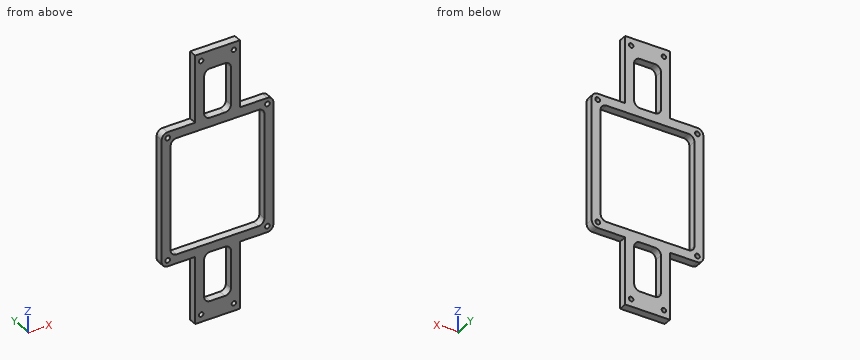
Autodesk Inventor part; units mm, degrees
ref_plane "YZ Plane" through (0, 0, 0) normal (1, 0, 0) x (0, 1, 0)
ref_plane "XZ Plane" through (0, 0, 0) normal (0, 1, 0) x (-1, 0, 0)
ref_plane "XY Plane" through (0, 0, 0) normal (0, 0, 1) x (1, 0, 0)
sketch "Sketch1" plane through (0, 0, 0) normal (0, 1, 0) x (-1, 0, 0)
  line L0 (37.5, 45) -> (-37.5, 45)
  line L1 (-37.5, 45) -> (-37.5, -45)
  line L2 (-37.5, -45) -> (37.5, -45)
  line L3 (37.5, -45) -> (37.5, 45)
  point P0 (0, 0)
  point P1 (37.5, 0)
  point P2 (0, 45)
  dimension "d0" = 90
  dimension "d1" = 75
extrude "Extrusion1" add sketch "Sketch1" along normal blind 5.334
sketch "Sketch2" plane through (0, 5.334, 0) normal (0, 1, 0) x (1, 0, 0)
  line L0 (-31.5, -39) -> (31.5, -39)
  line L1 (31.5, -39) -> (31.5, 39)
  line L2 (31.5, 39) -> (-31.5, 39)
  line L3 (-31.5, 39) -> (-31.5, -39)
  line L4 (-37.5, -45) -> (37.5, -45)
  line L5 (37.5, 45) -> (-37.5, 45)
  line L6 (-37.5, 45) -> (-37.5, -45)
  line L7 (37.5, -45) -> (37.5, 45)
  point P0 (0, 0)
  dimension "d4" = 6
  dimension "d5" = 6
  dimension "d6" = 6
  dimension "d7" = 6
extrude "Extrusion2" cut sketch "Sketch2" against normal through all contours L3 L2 L1 L0
sketch "Sketch3" plane through (0, 5.334, 0) normal (0, 1, 0) x (1, 0, 0)
  line L0 (-37.5, -45) -> (37.5, -45)
  line L1 (-37.5, 45) -> (-37.5, -45)
  line L2 (37.5, -45) -> (37.5, 45)
  line L3 (37.5, 45) -> (-37.5, 45)
  point P0 (0, 0)
  point P1 (-33.5, -41)
  point P2 (-33.5, 41)
  point P3 (33.5, 41)
  point P4 (33.5, -41)
  dimension "d10" = 4
  dimension "d11" = 4
  dimension "d12" = 4
  dimension "d13" = 4
hole "Hole1" at (-33.5, 5.334, 41) at (-33.5, 5.334, -41) at (33.5, 5.334, -41) at (33.5, 5.334, 41) direction (0, -1, 0) diameter 3.2 end through all
fillet "Fillet1" radius 4 8 edges at (-37.5, 2.667, 45) (-31.5, 2.667, 39) (37.5, 2.667, 45) (37.5, 2.667, -45) (31.5, 2.667, -39) (31.5, 2.667, 39) (-31.5, 2.667, -39) (-37.5, 2.667, -45)
sketch "Sketch4" plane through (33.5, 0, -45) normal (0, 0, -1) x (-1, 0, 0)
  line L0 (6, 5.334) -> (61, 5.334)
  line L1 (61, 0) -> (6, 0)
  line L2 (48.5, 5.334) -> (18.5, 5.334)
  line L3 (18.5, 5.334) -> (18.5, 0)
  line L4 (18.5, 0) -> (48.5, 0)
  line L5 (48.5, 0) -> (48.5, 5.334)
  point P0 (33.5, 0)
  dimension "d22" = 30
  dimension "d23" = 15
extrude "Extrusion3" add sketch "Sketch4" along normal blind 45
sketch "Sketch5" plane through (0, 5.334, 0) normal (0, 1, 0) x (1, 0, 0)
  line L0 (-15, 90) -> (15, 90)
  point P0 (0, 0)
  point P1 (-11, 85)
  point P2 (11, 85)
  dimension "d27" = 22
  dimension "d28" = 11
  dimension "d29" = 5
hole "Hole2" at (-11, 5.334, -85) at (11, 5.334, -85) direction (0, -1, 0) diameter 3 end through all
sketch "Sketch7" plane through (0, 5.334, 0) normal (0, 1, 0) x (1, 0, 0)
  line L0 (-5, 78) -> (5, 78)
  line L1 (9, 74) -> (9, 49)
  line L2 (5, 45) -> (-5, 45)
  line L3 (-9, 49) -> (-9, 74)
  arc A0 (-5, 78) -> (-9, 74) centre (-5, 74) ccw
  arc A1 (9, 74) -> (5, 78) centre (5, 74) ccw
  arc A2 (5, 45) -> (9, 49) centre (5, 49) ccw
  arc A3 (-9, 49) -> (-5, 45) centre (-5, 49) ccw
  line L4 (-15, 45) -> (-15, 90)
  line L5 (15, 45) -> (15, 90)
  line L6 (-15, 90) -> (15, 90)
  line L7 (33.5, 45) -> (15, 45)
  point P0 (0, 0)
  dimension "d43" = 4
  dimension "d44" = 6
  dimension "d45" = 6
  dimension "d46" = 12
extrude "Extrusion5" cut sketch "Sketch7" against normal through all
mirror "Mirror2" about plane through (0, 0, 0) normal (0, 0, 1) of "Extrusion3", "Extrusion5", "Hole2"
equation "\"d5\" = d4"
equation "\"d6\" = d4"
equation "\"d7\" = d4"
equation "\"d45\" = d44"
properties part number "phone_plate" material "Polycarbonate, Clear"
Build history of the part. All positions in model axes, mm. Coordinates: 2 decimals unless noted, no trailing zeros. Write each loop counter-clockwise with the first axis right and the second up, starting at its lowest first coordinate (ties: lowest second). Pieces come first, ordered by that corner, then holes.
1. Drill centre lines: probe 1 along Z at (x, y) = (-11, 3.5); probe 2 along Z at (x, y) = (33.5, 2.15); probe 3 along Z at (x, y) = (-1.5, 3.75). Where is each one in solid material? Low to high.
Answer block:
probe 1: z = -90 to -86.5, -83.5 to -39, 39 to 83.5, 86.5 to 90
probe 2: z = -45 to -42.6, -39.4 to 39.4, 42.6 to 45
probe 3: z = -90 to -78, -45 to -39, 39 to 45, 78 to 90
2. Band-saw the part on B-B, the plane y = 3.8. Give the number of separate pieces and of enclosed holes in the cut face, and give its area (3 significant figures).
Answer block:
separate pieces: 1
enclosed holes: 11
area: 3,320 mm2
3. Band-saw the part on A-A, the plane z = -4. Give the cut face in (x, y).
Answer block:
outline: (-37.5, 0) - (-31.5, 0) - (-31.5, 5.33) - (-37.5, 5.33) - close; (31.5, 0) - (37.5, 0) - (37.5, 5.33) - (31.5, 5.33) - close
4. Drop flat-ended pins along their axis: pin 1 (3.5 mm diameter, centred on x = 11, z = 85, fed in from +Y); pin 2 (1 mm diameter, centred on y = 1.5, z = 50, fed in from +X); pin 3 (2 mm diameter, centred on x = 29.5, y = 3, fed in from +Z); pin 4 (1.6 mm diameter, centred on x = -23.5, y = 4, fed in from -Z). Give the stop position or say it passes through.
Answer block:
pin 1: stops at y = 5.33
pin 2: stops at x = 15
pin 3: stops at z = 45
pin 4: stops at z = -45
